Can you work these out from the model? Positions are in its coordinate system, mm. Face numbers are marked on the shaded views. Round coordinates to 2 decimals unless told otherwise and drop trailing zeros. Write each loop counter-clockwise with the first axis right and the second up, starting at its lowest first coordinate (ties: lowest second). Pieces come first, ordered by that corner, then holes. Notation, with made-up numbers: (-5.5, 36.25) - (25.5, 36.25) arc R8 ccw to (25.5, 41.25) - close; hole circle Ø7 at (-32, 44.5). An arc over 180 degrees is marked (long way). One line per item, written item: value. Start each with the question number.
(1) I want a section at D-D on x = 31.75. List the corners of the cut face in (y, z) for me (3 decimals).
(2) If I drill on L1, parallel to X at y = -26, z = 5.75; L2, parallel to X at y = -30.5, z = 5.5; L3, parallel to Y at x = -31.75, z = 5 (3 decimals), over which ranges is the centre line in solid material (lowest first)? Write a range as from..to.
(3) Thinking about a two-plate mould opening in X: for the marked faces 1 and 2, which applies, +X half, -X half, draft (parallel to the pull), parting line (faces both ways), or undercut?
(4) I'm going to push flat-ended pins straight in: pin 1 Ø5 at (x, y) = (39, -8.5) entering from -Z; pin 2 Ø3 at (y, z) = (-37, 3) entering from -X; pin 3 Ø2 at (x, z) = (28, 4.5) entering from -Y; pin 4 Ø2 at (y, z) = (-19, 4) entering from -X. Where does each tip first touch, or does it pass through?
(5) I want a section at C-C on z = 4.5. List the corners of the cut face in (x, y) for me (3 decimals).
(6) I want a section at B-B on x = 0. List the corners of the cut face in (y, z) for me (3 decimals), plus the area to 3 significant figures.
(7) I want a section at A-A on x = 12.7. List the corners of the cut face in (y, z) for me (3 decimals), plus the area to 3 significant figures.
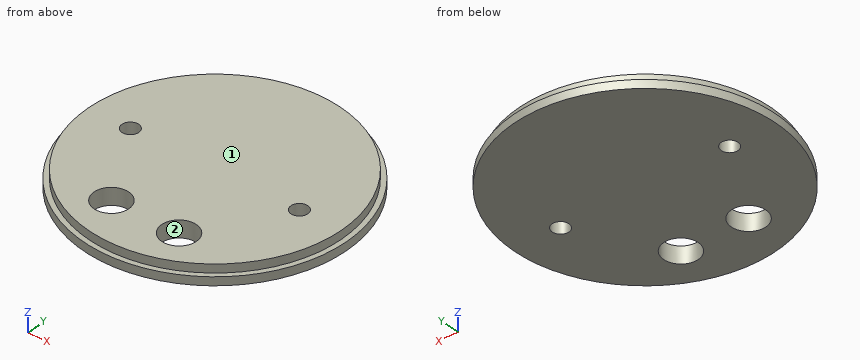
from build123d import *

# Parameters (mm, degrees)
SKETCH1_R           = 49.5046
BOSS_EXTRUDE1_DEPTH = 3.175
SKETCH2_R           = 47.625
BOSS_EXTRUDE2_DEPTH = 3.175
SKETCH3_R           = 6.5484375
SKETCH3_R_2         = 3.175
CUT_EXTRUDE1_DEPTH  = 7.35


with BuildPart() as part:
    # Sketch1 → Boss-Extrude1 (new body)
    with BuildSketch(Plane.XY):
        Circle(SKETCH1_R)
    extrude(amount=BOSS_EXTRUDE1_DEPTH)

    # Sketch2 → Boss-Extrude2 (add)
    with BuildSketch(Plane.XY.offset(3.175)):
        Circle(SKETCH2_R)
    extrude(amount=BOSS_EXTRUDE2_DEPTH)

    # Sketch3 → Cut-Extrude1 (cut, through all)
    with BuildSketch(Plane.XY.offset(6.35)):
        with Locations((-12.7, -31.166793627)):
            Circle(SKETCH3_R)
        with Locations((12.7, -31.166793627)):
            Circle(SKETCH3_R)
        with Locations((-31.75, 0)):
            Circle(SKETCH3_R_2)
        with Locations((31.75, 0)):
            Circle(SKETCH3_R_2)
    extrude(amount=-CUT_EXTRUDE1_DEPTH, mode=Mode.SUBTRACT)


solid = part.part
Established:
1. outline: (-37.982, 0) - (-3.175, 0) - (-3.175, 6.35) - (-35.498, 6.35) - (-35.498, 3.175) - (-37.982, 3.175) - close; (3.175, 0) - (37.982, 0) - (37.982, 3.175) - (35.498, 3.175) - (35.498, 6.35) - (3.175, 6.35) - close
2. L1: -39.9..-16.72, -8.68..8.68, 16.72..39.9
2. L2: -36.58..-19.21, -6.19..6.19, 19.21..36.58
2. L3: -35.498..-3.175, 3.175..35.498
3. face 1: draft
3. face 2: undercut
4. pin 1: z = 0
4. pin 2: x = -34.5
4. pin 3: y = -39.23
4. pin 4: x = -45.94
5. outline: circle Ø95.25 at (0, 0); hole circle Ø6.35 at (-31.75, 0); hole circle Ø13.097 at (-12.7, -31.167); hole circle Ø13.097 at (12.7, -31.167); hole circle Ø6.35 at (31.75, 0)
6. outline: (-49.505, 0) - (49.505, 0) - (49.505, 3.175) - (47.625, 3.175) - (47.625, 6.35) - (-47.625, 6.35) - (-47.625, 3.175) - (-49.505, 3.175) - close
6. area: 617 mm2
7. outline: (-47.848, 0) - (-37.715, 0) - (-37.715, 6.35) - (-45.9, 6.35) - (-45.9, 3.175) - (-47.848, 3.175) - close; (-24.618, 0) - (47.848, 0) - (47.848, 3.175) - (45.9, 3.175) - (45.9, 6.35) - (-24.618, 6.35) - close
7. area: 512 mm2
